Check sheet for the modelled part. Datum: model origin and axes. Units: mm. A direction names the side the tool comes from. Round coordinates to 2 decimals unless told otherwise and drop trailing zeros. Write each loop counter-clockwise with the first axis right and the second up, starting at its lowest first coordinate (ties: lowest second). Pieces come first, ordered by that corner, then holes. Notation, with made-up numbers: (-24, -31.5) - (34, -31.5) arc R13 ccw to (34, -17.5) - close; hole circle Ø2 at (-16, 79). An arc over 180 degrees is marked (long way). Answer as a JSON object with one key per item and string values. Group by question number.
Item 1: Release check for a two-part mould opening along X. For faces 4 (the flat face through (-114, 0, 50)), 5 (the flat face through (-50.09, -50.09, 64.03)), 6 (the flat face through (-127, -50, 52)) record: pulls with the +X half, pulls with the -X half, needs draft (parallel to the pull), parting line crosses it, or undercut.
Item 2: Set-up check for faces 1 (the flat face through (-114, -101.308, 50)), 2 (the flat face through (13, -52, 101.6)), 3 (the flat face through (0, -63, 73)): record each of +Z, -Z, +X, -X, +Y, -Y from which the full face is reachable in a straight line by a thin tool's end or side.
Item 3: Sectioned sample at C-C on x = -88.5. Record the boundary of the cut face in (y, z), plus the area to 3 significant figures.
Item 4: Sectioned sample at D-D on z = 38.5. Record the boundary of the cut face in (x, y).
Item 5: Thickness scan on line 1 (X direction, y = -81, z = 97); line 2 (Y direction, x = -116.5, z = 54); line 3 (Z direction, x = 9.5, y = -38). Record the ranges inside material, lowest first.
Item 6: Sectioned sample at A-A on z = 27.5. Record the boundary of the cut face in (x, y), plus the area to 3 significant figures.
Item 7: Sectioned sample at B-B on y = -16. Record the boundary of the cut face in (x, z).
Item 8: Gauge pin test, flat ends, axial feed: P1, Ø6, axis at x = -78, z = 82, coming from the -Y side; P2, Ø12.5, axis at x = -119.5, z = 34, coming from the -Y side; P3, Ø8, axis at x = -66, z = 51, coming from the -Y side. Record the tip position at first contact, or that the pin passes through.
```python
from build123d import *

# Parameters (mm, degrees)
F0_W     = 101.6
F0_H     = 101.6
F1_DEPTH = 25.4
F3_DEPTH = 101.6
F4_W     = 101.6
F4_H     = 101.6
F5_DEPTH = 25.4
F6_W     = 101.307563
F6_H     = 102.009408
F7_DEPTH = 25.4


with BuildPart() as f1:
    # F0 (on Top) → F1 (new body)
    with BuildSketch(Plane.XY):
        with Locations((-50.8, -50.8)):
            Rectangle(F0_W, F0_H)
    extrude(amount=F1_DEPTH)

    # F2 (on face) → F3 (join)
    with BuildSketch(Plane.YZ):
        Polygon((-101.6, 25.4), (0, 25.4), (0, 101.6), align=None)
    extrude(amount=-F3_DEPTH)

    # F4 (on face) → F5 (join)
    with BuildSketch(Plane.YZ):
        with Locations((-50.8, 50.8)):
            Rectangle(F4_W, F4_H)
    extrude(amount=F5_DEPTH)

    # F6 (on face) → F7 (join)
    with BuildSketch(Plane(origin=(-101.6, 0, 0), x_dir=(0, -1, 0), z_dir=(-1, 0, 0))):
        with Locations((50.653782, 51.004704)):
            Rectangle(F6_W, F6_H)
    extrude(amount=F7_DEPTH)


solid = f1.part
```
Completed:
{
 "1": {"face 4": "needs draft", "face 5": "undercut", "face 6": "pulls with the -X half"},
 "2": {"face 1": "+Z, -Z, -X, -Y", "face 2": "+Z, +X, +Y, -Y", "face 3": "+Z, -Y"},
 "3": {"outline": "(-101.6, 0) - (0, 0) - (0, 101.6) - (-101.6, 25.4) - close", "area": "6,450 mm²"},
 "4": {"outline": "(-127, -101.31) - (-101.6, -101.31) - (-101.6, -84.13) - (0, -84.13) - (0, -101.6) - (25.4, -101.6) - (25.4, 0) - (-127, 0) - close"},
 "5": {"line 1": "-127 to -101.6, 0 to 25.4", "line 2": "-101.31 to 0", "line 3": "0 to 101.6"},
 "6": {"outline": "(-127, -101.31) - (-101.6, -101.31) - (-101.6, -98.8) - (0, -98.8) - (0, -101.6) - (25.4, -101.6) - (25.4, 0) - (-127, 0) - close", "area": "15,200 mm²"},
 "7": {"outline": "(-127, 0) - (25.4, 0) - (25.4, 101.6) - (0, 101.6) - (0, 89.6) - (-101.6, 89.6) - (-101.6, 102.01) - (-127, 102.01) - close"},
 "8": {"P1": "y = -30.13", "P2": "y = -101.31", "P3": "y = -72.8"}
}
